Can you work these out from the model? Positions are in its coordinate system, mm. A direction names the side the tool comes from. Coordinates: 2 decimals unless noted, no trailing zeros. Write each loop counter-clockwise with the first axis right and the second up, starting at its lowest first coordinate (ties: lowest second). Pieces come first, ordered by that corner, then holes. Notation, with made-up numbers: (10.25, 64) - (40.25, 64) arc R22 ccw to (40.25, 94) - close; hole circle Ø4 at (46.5, 13.5). An arc over 180 degrees is marked (long way). Use one line per item in the form item = value. Start each with the question number.
(1) Thinking about a two-plate mould opening in Y: for faces 1 (the face through (10, 2, 14)), 2 (the face through (99, 44, 3)), 3 (the face through (31.687, 37.815, 1.479)), which applies, pulls with the +Y half, pulls with the -Y half, needs draft (parallel to the pull), parting line crosses it, or undercut?
(2) On a 3-axis mill with a long thin cutter (end or side, diameter ignored), from which of +Z, -Z, +X, -X, +Y, -Y can I reach the whole of each face in a straight line? I mean faces 4 (the face through (124.81, 91.23, 5.46)), 5 (the face through (190, 2, 14)), 6 (the face through (81.4, 36.6, 8)). Say none if no direction works.
(3) If I drill on probe 1 along Y at (x, z) = (108, 6.3); probe 2 along Y at (x, z) = (75, 6.9); probe 3 along Z at (x, y) = (124.5, 13), over which ranges is the centre line in solid material (lowest first)? Write a range as from..to.
(4) If we section it at C-C on y = 9: Please give me the cut outline in (x, z).
(5) If we section it at B-B on y = 83.5: Please give me the cut outline in (x, z), then the cut area to 3 significant figures.
(6) For pin 1 Ø3.5 at (x, y) = (122.5, 89) entering from +Z; pin 2 Ø1.8 at (x, y) = (123.2, 88.7) entering from +Z; pin 3 Ø1.5 at (y, z) = (79.5, 1) entering from -X; pin 4 Ø12 at (x, z) = (134.5, 15.5) entering from -Y, each with a flat end and sliding along its axis, tell me the tip position at first contact or that it passes through.
(7) If we section it at A-A on x = 171: Please give me the cut outline in (y, z).
```python
from build123d import *

# Parameters (mm, degrees)
PAD_DEPTH       = 3
PAD001_DEPTH    = 5
SKETCH002_R     = 1.6
POCKET_DEPTH    = 100.001
SKETCH003_R     = 3
SKETCH003_R_2   = 1.5
PAD002_DEPTH    = 5
CHAMFER_SIZE    = 3
CHAMFER001_SIZE = 2


with BuildPart() as part:
    # Sketch → Pad (new body)
    with BuildSketch(Plane.XY):
        Polygon((0, 0), (200, 0), (200, 15), (137.5, 60), (137.5, 100), (62.5, 100), (62.5, 60), (0, 15), align=None)
    extrude(amount=PAD_DEPTH)

    # Sketch001 (on Face1 of Pad) → Pad001 (join)
    with BuildSketch(Plane.XZ):
        Polygon((0, 3), (0, 20), (10, 20), (10, 7.5), (190, 7.5), (190, 20), (200, 20), (200, 3), align=None)
    extrude(amount=-PAD001_DEPTH)

    # Sketch002 (on Face14 of Pad001) → Pocket (cut, through all)
    with BuildSketch(Plane.XZ):
        with Locations((7.5, 7.5)):
            Circle(SKETCH002_R)
        with Locations((192.5, 7.5)):
            Circle(SKETCH002_R)
    extrude(amount=-POCKET_DEPTH, mode=Mode.SUBTRACT)

    # Sketch003 (on Face7 of Pocket) → Pad002 (join)
    with BuildSketch(Plane.XY.offset(3)):
        with Locations((75, 90)):
            Circle(SKETCH003_R)
        with Locations((75, 90)):
            Circle(SKETCH003_R_2, mode=Mode.SUBTRACT)
        with Locations((123.2, 88.7)):
            Circle(SKETCH003_R)
        with Locations((123.2, 88.7)):
            Circle(SKETCH003_R_2, mode=Mode.SUBTRACT)
        with Locations((108, 37.9)):
            Circle(SKETCH003_R)
        with Locations((108, 37.9)):
            Circle(SKETCH003_R_2, mode=Mode.SUBTRACT)
        with Locations((80.1, 37.9)):
            Circle(SKETCH003_R)
        with Locations((80.1, 37.9)):
            Circle(SKETCH003_R_2, mode=Mode.SUBTRACT)
    extrude(amount=PAD002_DEPTH)

    # Chamfer
    chamfer_edges = [part.edges().sort_by_distance(p)[0] for p in [
        (10, 2.5, 7.5),
        (190, 2.5, 7.5),
        (190, 2.5, 20),
        (10, 2.5, 20),
    ]]
    chamfer(chamfer_edges, length=CHAMFER_SIZE)

    # Chamfer001
    chamfer001_edges = [part.edges().sort_by_distance(p)[0] for p in [
        (100, 5, 3),
    ]]
    chamfer(chamfer001_edges, length=CHAMFER001_SIZE)


solid = part.part
```
Reported:
q1.face_1 = needs draft
q1.face_2 = undercut
q1.face_3 = pulls with the +Y half
q2.face_4 = +Z
q2.face_5 = +Z, +Y, -Y
q2.face_6 = +Z, +X, -X, +Y, -Y
q3.probe_1 = 0..5, 34.9..36.4, 39.4..40.9
q3.probe_2 = 0..5, 87..88.5, 91.5..93
q3.probe_3 = 0..3
q4.outline = (0, 0) - (200, 0) - (200, 3) - (0, 3) - close
q5.outline = (62.5, 0) - (137.5, 0) - (137.5, 3) - (62.5, 3) - close
q5.area = 225 mm2
q6.pin_1 = 8
q6.pin_2 = 3
q6.pin_3 = 62.5
q6.pin_4 = through
q7.outline = (0, 0) - (35.88, 0) - (35.88, 3) - (7, 3) - (5, 5) - (5, 7.5) - (0, 7.5) - close
